Study the drawing (mm; zero at the part's minimum x, y, z) and answer. Coordinates: 2 decimals unless noted, no trailing zeros. Loops run counter-clockwise (first coordinate to the right, second up) from the corner with the lowest first, then second, coordinate; pieces in that order, holes last. Notation, with made-up numbers: (81.25, -1) -> (138.25, -1) arc R21 ccw to (138.25, 18) -> close; hole circle Ø10 at (86, 84). An arc over 180 degrees is marked (long way). Answer in a Markdown table with one row per item.
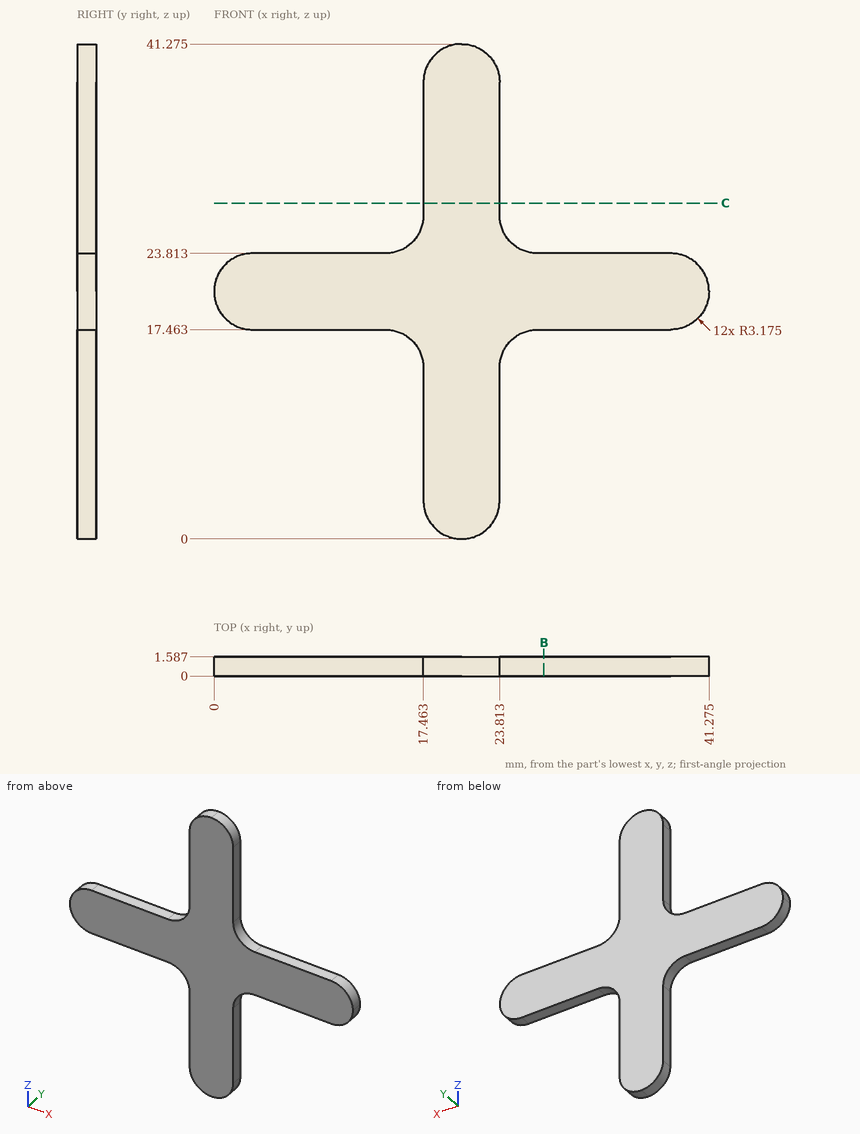
1. A cutting plane is placed at C-C on z = 28. Give the vertices of the cut face in (x, y), and give its area (3 significant figures).
A:
| item | result |
|---|---|
| outline | (17.46, 0) -> (23.81, 0) -> (23.81, 1.59) -> (17.46, 1.59) -> close |
| area | 10.1 mm2 |
2. Given pin 1 Ø0.5 at (y, z) = (0.5, 31.5) entering from +X; pin 2 Ø0.5 at (x, y) = (33, 0.5) entering from -Z, each flat-ended and moving along its own axis, determine where each tip first touches the part or whether it passes through.
A:
| item | result |
|---|---|
| pin 1 | stops at x = 23.81 |
| pin 2 | stops at z = 17.46 |
3. A cutting plane is placed at B-B on x = 27.5. Give the vertices of the cut face in (y, z).
A:
| item | result |
|---|---|
| outline | (0, 17.46) -> (1.59, 17.46) -> (1.59, 23.81) -> (0, 23.81) -> close |
4. Find the intervals of material crossed by probe 1 along Z at (x, y) = (29, 1); probe 2 along X at (y, z) = (0.6, 25) (1 decimal), in increasing order.
A:
| item | result |
|---|---|
| probe 1 | z = 17.46 to 23.81 |
| probe 2 | x = 16.8 to 24.5 |
